Source: CAD feature listing. Evaluate the final solid. Frame: model axes, mm. A direction names the side the tool comes from. Coordinates: 2 decimals unless noted, no trailing zeros. Write each loop counter-clockwise with the first axis right and the second up, starting at its lowest first coordinate (ties: lowest second). Pieces come first, ordered by that corner, then holes. Notation, with made-up numbers: (67.25, -9.5) -> (108.25, -9.5) arc R14 cw to (108.25, 7.5) -> close; hole circle Ø10 at (-4, 13). An arc over 180 degrees is marked (long way). One line per item, written item: value. Start each with the question number.
1. Mould query, pull axis Y, two halves, no side actions, for faces 1 (the cylindrical face through (12.633, 29.815, -0.112)), 2 (the flat face through (-9, -18, -8)), 3 (the flat face through (0, 40, 0)). Classes: released by +Y, released by -Y, zero draft, split by the parting line, or undercut.
2. Section query C-C, the plane z = 4.25. Output: boundary loops of the cut face in (x, y), and give its area (3 significant figures).
3. Line query: line 1 (Z direction, x = -37.5, y = -35.5); line 2 (Y direction, x = -0.5, z = 0.5); line 3 (X direction, y = -34, z = -1.5). Output: solid intervals per line, ascending.
4. Section query A-A, the plane y = 10. Output: boundary loops of the cut face in (x, z), and give its area (3 significant figures).
5. Section query B-B, the plane x = -37.5. Output: boundary loops of the cut face in (y, z), and give its area (3 significant figures).
6. Access query for faces 4 (the flat face through (30, 5, 0)), 5 (the flat face through (-34, -30, 0)), 6 (the flat face through (-45, -35, 0)). Directions: +Z, -Z, +X, -X, +Y, -Y. A direction counts if a zero-diameter tool reaches every point of the face in a straight line with its end or side. Return the directions, or none.
7. First-contact query: P1, Ø8, axis at y = 4, z = -3.5, coming from the +X side; P2, Ø1.5, axis at x = -34.5, z = -6, coming from the +Y side; P3, Ø3, axis at y = -6, z = -3, coming from the -X side. Flat tips, straight axial feed; report the tip coordinate or a pass-through.
8. Section query D-D, the plane y = 34.5. Output: boundary loops of the cut face in (x, z), and give its area (3 significant figures).
from build123d import *

# Parameters (mm, degrees)
SKETCH1_W           = 60
SKETCH1_H           = 80
SKETCH1_R           = 23.5
BOSS_EXTRUDE1_DEPTH = 8
SKETCH2_W           = 15
SKETCH2_H           = 16
SKETCH2_R           = 3.25
BOSS_EXTRUDE2_DEPTH = 10


with BuildPart() as part:
    # Sketch1 → Boss-Extrude1 (new body, symmetric)
    with BuildSketch(Plane.XY):
        Rectangle(SKETCH1_W, SKETCH1_H)
        with Locations((0, 10)):
            Circle(SKETCH1_R, mode=Mode.SUBTRACT)
    extrude(amount=BOSS_EXTRUDE1_DEPTH, both=True)

    # Sketch2 → Boss-Extrude2 (add)
    with BuildSketch(Plane.XZ.offset(40)):
        with Locations((37.5, 0)):
            Rectangle(SKETCH2_W, SKETCH2_H)
        with Locations((37.5, 0)):
            Circle(SKETCH2_R, mode=Mode.SUBTRACT)
    boss_extrude2 = extrude(amount=-BOSS_EXTRUDE2_DEPTH)

    # Mirror1: Boss-Extrude2 across plane
    add(boss_extrude2.mirror(Plane(origin=(0, 0, 0), x_dir=(0, 0, 1), z_dir=(1, 0, 0))))


solid = part.part
Computed values:
1. face 1: undercut
1. face 2: zero draft
1. face 3: released by +Y
2. outline: (-45, -40) -> (45, -40) -> (45, -30) -> (30, -30) -> (30, 40) -> (-30, 40) -> (-30, -30) -> (-45, -30) -> close; hole circle Ø47 at (0, 10)
2. area: 3,370 mm²
3. line 1: z = -8 to -3.25, 3.25 to 8
3. line 2: y = -40 to -13.49, 33.49 to 40
3. line 3: x = -45 to -40.38, -34.62 to 34.62, 40.38 to 45
4. outline: (-30, -8) -> (-23.5, -8) -> (-23.5, 8) -> (-30, 8) -> close; (23.5, -8) -> (30, -8) -> (30, 8) -> (23.5, 8) -> close
4. area: 208 mm²
5. outline: (-40, -8) -> (-30, -8) -> (-30, -3.25) -> (-40, -3.25) -> close; (-40, 3.25) -> (-30, 3.25) -> (-30, 8) -> (-40, 8) -> close
5. area: 95.0 mm²
6. face 4: +Z, -Z, +X, +Y
6. face 5: +Z, -Z, -X, +Y
6. face 6: +Z, -Z, -X, +Y, -Y
7. P1: stops at x = 30
7. P2: stops at y = -30
7. P3: stops at x = -30
8. outline: (-30, -8) -> (30, -8) -> (30, 8) -> (-30, 8) -> close
8. area: 960 mm²
